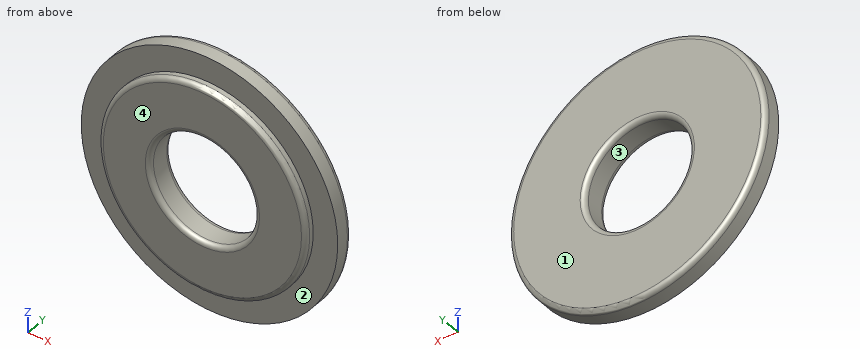
```python
from build123d import *

# Parameters (mm, degrees)
SKETCH1_R           = 28.2575
BOSS_EXTRUDE1_DEPTH = 2.54
SKETCH2_R           = 34.925
BOSS_EXTRUDE2_DEPTH = 4.7625
CUT_EXTRUDE1_REACH  = 9.303
SKETCH3_R           = 14.2875
FILLET1_R           = 1.27


with BuildPart() as part:
    # Sketch1 → Boss-Extrude1 (new body)
    with BuildSketch(Plane(origin=(0, 0, 0), x_dir=(1, 0, 0), z_dir=(0, 1, 0))):
        Circle(SKETCH1_R)
    extrude(amount=BOSS_EXTRUDE1_DEPTH)

    # Sketch2 → Boss-Extrude2 (add)
    with BuildSketch(Plane(origin=(0, 2.54, 0), x_dir=(1, 0, 0), z_dir=(0, 1, 0))):
        Circle(SKETCH2_R)
    extrude(amount=BOSS_EXTRUDE2_DEPTH)

    # Sketch3 → Cut-Extrude1 (cut, up to next)
    with BuildSketch(Plane.XZ, mode=Mode.PRIVATE) as cut_extrude1_sk1:
        Circle(SKETCH3_R)
    cut_extrude1_tool1 = extrude(cut_extrude1_sk1.sketch, amount=-CUT_EXTRUDE1_REACH, mode=Mode.PRIVATE) & part.part
    add(cut_extrude1_tool1.solids().sort_by_distance((0, 0, 0))[0], mode=Mode.SUBTRACT)

    # Fillet1
    fillet1_edges = [part.edges().sort_by_distance(p)[0] for p in [
        (-14.2875, 7.3025, 0),
        (-14.2875, 0, 0),
        (-28.2575, 0, 0),
        (-34.925, 7.3025, 0),
    ]]
    fillet(fillet1_edges, radius=FILLET1_R)


solid = part.part
```
Check sheet for the modelled part. Datum: model origin and axes. Units: mm. Face numbers are marked on the shaded views. A direction names the side the tool comes from. Give positions to 0.01 mm unless a question says otherwise; leave off trailing zeros. Write each loop counter-clockwise with the first axis right and the second up, starting at its lowest first coordinate (ties: lowest second). Pieces come first, ordered by that corner, then holes. Notation, with made-up numbers: (-17, 13) -> (1, 13) arc R16 ccw to (1, 19) -> close; hole circle Ø1 at (-2.5, 60.25). An arc over 180 degrees is marked (long way). Use CSV: the item, a comma, the result in double quotes. Start each with the question number.
Q1. Scan lines: line 1 along Z through (x, y) = (0, 2.35); line 2 along Z through (x, y) = (0, 2.65) (1 decimal); line 3 along Y through (x, z) = (10.5, 27). Record each from-to range of solid material in increasing order.
Q2. Depth check by flat-ended pin: P1, Ø1.5, axis at x = -20, y = 2, coming from the +Z side; P2, Ø1.5, axis at x = -1.5, y = 1.5, coming from the +Z side; P3, Ø1, axis at x = 12, y = 5, coming from the -Z side. Enter the tip coordinate at first touch or a pass-through.
Q3. Cross-section at A-A on z = 0. Enter the section's corners in (x, y) (1 decimal), and give its area (3 significant figures).
Q4. Tool access check on the marked faces 1 and 2. Record the directions out of +Z, -Z, +X, -X, +Y, -Y that give a thin tool (end or side, any length) a straight path to the whole face; none if there is none.
Q5. Release check for a two-part mould opening along Z. For the marked faces 3 and 4 record: +Z half, -Z half, draft (parallel to the pull), parting line (faces both ways), or undercut.
Q6. Cross-section at B-B on x = 0. Enter the section's corners in (y, z) (1 decimal).
Working result:
1,line 1,"z = -28.26 to -14.29, 14.29 to 28.26"
1,line 2,"z = -34.9 to -14.3, 14.3 to 34.9"
1,line 3,"y = 2.54 to 7.3"
2,P1,"stops at z = 28.99"
2,P2,"stops at z = 28.25"
2,P3,"stops at z = -32.98"
3,outline,"(-34.9, 2.5) -> (-28.3, 2.5) -> (-28.3, 1.3) arc R1.3 ccw to (-27, 0) -> (-15.6, 0) arc R1.3 ccw to (-14.3, 1.3) -> (-14.3, 6) arc R1.3 ccw to (-15.6, 7.3) -> (-33.7, 7.3) arc R1.3 ccw to (-34.9, 6) -> close; (14.3, 1.3) arc R1.3 ccw to (15.6, 0) -> (27, 0) arc R1.3 ccw to (28.3, 1.3) -> (28.3, 2.5) -> (34.9, 2.5) -> (34.9, 6) arc R1.3 ccw to (33.7, 7.3) -> (15.6, 7.3) arc R1.3 ccw to (14.3, 6) -> close"
3,area,"265 mm^2"
4,face 1,"+Z, -Z, +X, -X, +Y"
4,face 2,"-Y"
5,face 3,"undercut"
5,face 4,"draft"
6,outline,"(0, -27) arc R1.3 ccw to (1.3, -28.3) -> (2.5, -28.3) -> (2.5, -34.9) -> (6, -34.9) arc R1.3 ccw to (7.3, -33.7) -> (7.3, -15.6) arc R1.3 ccw to (6, -14.3) -> (1.3, -14.3) arc R1.3 ccw to (0, -15.6) -> close; (0, 15.6) arc R1.3 ccw to (1.3, 14.3) -> (6, 14.3) arc R1.3 ccw to (7.3, 15.6) -> (7.3, 33.7) arc R1.3 ccw to (6, 34.9) -> (2.5, 34.9) -> (2.5, 28.3) -> (1.3, 28.3) arc R1.3 ccw to (0, 27) -> close"
